```python
from build123d import *

# Parameters (mm, degrees)
F0_W     = 127
F0_H     = 85.5306185286
F1_DEPTH = 254
F2_W     = 44.157743454
F2_H     = 12.9875717685
F3_DEPTH = 76.2
F4_W     = 12.6961972564
F4_H     = 7.905177772
F5_DEPTH = 12.7
F6_W     = 9.1298371553
F6_H     = 11.8159283884
F6_W_2   = 8.5927993059
F6_H_2   = 6.6836136393
F6_W_3   = 35.9823405743
F7_DEPTH = 76.2


with BuildPart() as f1:
    # F0 (on Front) → F1 (new body)
    with BuildSketch(Plane.XZ):
        with Locations((-1.4842953533, -1.855365932)):
            Rectangle(F0_W, F0_H)
    extrude(amount=F1_DEPTH)

    # F2 (on Right) → F3 (join)
    with BuildSketch(Plane.YZ):
        Polygon((-157.0569574833, 18.924748525), (-212.3468965292, 18.924748525), (-212.3468965292, -15.9561578184), (-168.9313054085, -15.9561578184), (-168.9313054085, 0), (-157.0569574833, 0), align=None)
        Polygon((-108.4463298321, 0), (-157.0569574833, 18.924748525), (-157.0569574833, 0), align=None)
        Polygon((-168.9313054085, -15.9561578184), (-212.3468965292, -15.9561578184), (-168.9313054085, -32.6544642448), align=None)
        Polygon((-108.4463298321, 0), (-157.0569574833, 0), (-157.0569574833, -15.9561578184), (-168.9313054085, -15.9561578184), (-168.9313054085, -32.6544642448), (-108.4463298321, -32.6544642448), (-108.4463298321, -21.8933336437), (-116.9810146093, -21.8933336437), (-116.9810146093, -8.9057618752), (-108.4463298321, -8.9057618752), align=None)
        Polygon((-64.2885863781, -8.9057618752), (-108.4463298321, 0), (-108.4463298321, -8.9057618752), align=None)
        with Locations((-86.3674581051, -15.3995477594)):
            Rectangle(F2_W, F2_H)
        Polygon((-108.4463298321, -21.8933336437), (-108.4463298321, -32.6544642448), (-64.2885863781, -21.8933336437), align=None)
    extrude(amount=F3_DEPTH)

    # F4 (on Front) → F5 (join)
    with BuildSketch(Plane.XZ):
        Polygon((-24.3036681507, 11.0724206409), (-24.1946410388, 11.0193416476), (11.4984409884, 11.0193416476), (11.4984409884, 25.6319474429), align=None)
        Polygon((11.4984409884, 11.0193416476), (-24.1946410388, 11.0193416476), (-24.1946410388, 9.8215872422), (-16.5290106088, 9.8215872422), (-16.5290106088, 2.1559579764), (-24.1946410388, 2.1559579764), (-24.1946410388, -17.2476638108), (-18.684970215, -17.2476638108), (-7.1865268983, -17.2476638108), (-7.1865268983, -10.779789649), (19.6431726217, -10.779789649), (19.6431726217, 0), (11.4984409884, 0), align=None)
        Polygon((-24.1946410388, 9.8215872422), (-24.1946410388, 11.0193416476), (-24.3036681507, 11.0724206409), (-42.400509119, 19.8827255517), (-42.400509119, 9.8215872422), align=None)
        Polygon((11.4984409884, 25.6319474429), (11.4984409884, 11.0193416476), (19.6431726217, 11.0193416476), (19.6431726217, 0), (48.6288368702, 0), (48.6288368702, 25.6319474429), align=None)
        Polygon((-24.1946410388, 2.1559579764), (-24.1946410388, 9.8215872422), (-42.400509119, 9.8215872422), (-42.400509119, 7.186527364), (-45.2751219273, 7.186527364), (-45.2751219273, 2.1559579764), (-41.9214069843, 2.1559579764), (-41.9214069843, 4.072365351), (-29.4647607952, 4.072365351), (-29.4647607952, 2.1559579764), align=None)
        Polygon((-24.1946410388, -17.2476638108), (-24.1946410388, 2.1559579764), (-29.4647607952, 2.1559579764), (-29.4647607952, -4.3119159527), align=None)
        Polygon((-45.2751219273, 9.8215872422), (-42.400509119, 9.8215872422), (-42.400509119, 19.8827255517), (-57.9713173211, 19.8827255517), (-57.9713173211, 7.186527364), (-45.2751219273, 7.186527364), align=None)
        Polygon((48.6288368702, 0), (19.6431726217, 0), (19.6431726217, -10.779789649), (31.6207185388, -10.779789649), (31.6207185388, -5.5096708238), (47.6706326008, -5.5096708238), align=None)
        Polygon((-41.9214069843, -12.6961972564), (-24.1946410388, -17.2476638108), (-29.4647607952, -4.3119159527), (-29.4647607952, -12.6961972564), align=None)
        Polygon((-29.4647607952, -4.3119159527), (-29.4647607952, 2.1559579764), (-41.9214069843, 2.1559579764), (-41.9214069843, -12.6961972564), (-29.4647607952, -12.6961972564), align=None)
        Polygon((31.6207185388, -10.779789649), (19.6431726217, -10.779789649), (19.6431726217, -17.2476638108), (-7.1865268983, -17.2476638108), (-7.1865268983, -32.3393717408), (9.5820333809, -32.3393717408), (9.5820333809, -25.3923945129), (22.2782306373, -25.3923945129), (22.2782306373, -32.3393717408), (29.2252078652, -32.3393717408), (35.6930866838, -32.3393717408), (35.6930866838, -24.6737431735), (31.6207185388, -24.6737431735), align=None)
        Polygon((-7.1865268983, -17.2476638108), (-18.684970215, -17.2476638108), (-7.1865268983, -32.3393717408), align=None)
        Polygon((-45.2751219273, 2.1559579764), (-41.9214069843, -12.6961972564), (-41.9214069843, 2.1559579764), align=None)
        Polygon((-45.2751219273, 2.1559579764), (-45.2751219273, 7.186527364), (-57.9713173211, 7.186527364), align=None)
        Polygon((31.6207185388, -5.5096708238), (31.6207185388, -10.779789649), (35.6930866838, -10.779789649), (35.6930866838, -24.6737431735), (47.6706326008, -24.6737431735), (47.6706326008, -5.5096708238), align=None)
        Polygon((9.5820333809, -32.3393717408), (-7.1865268983, -32.3393717408), (9.5820333809, -40.2445495129), align=None)
        Polygon((35.6930866838, -32.3393717408), (47.6706326008, -24.6737431735), (35.6930866838, -24.6737431735), align=None)
        with Locations((15.9301320091, -36.2919606268)):
            Rectangle(F4_W, F4_H)
        Polygon((29.2252078652, -32.3393717408), (22.2782306373, -32.3393717408), (22.2782306373, -40.2445495129), align=None)
    extrude(amount=-F5_DEPTH)

    # F6 (on Right) → F7 (join)
    with BuildSketch(Plane.YZ):
        Polygon((-38.9934703708, -82.4129879475), (-38.9934703708, 11.0402805731), (-61.0125139356, 11.0402805731), (-61.0125139356, -6.6836136393), (-52.4197183549, -6.6836136393), (-52.4197183549, -29.7783855349), (-61.0125139356, -29.7783855349), (-61.0125139356, -82.4129879475), align=None)
        Polygon((-18.666213934, -19.4484525669), (-38.9934703708, 11.0402805731), (-38.9934703708, -82.4129879475), align=None)
        Polygon((-61.0125139356, 11.0402805731), (-38.9934703708, 11.0402805731), (-8.3816275001, 31.4496159554), align=None)
        Polygon((-61.0125139356, -6.6836136393), (-61.0125139356, 11.0402805731), (-137.8106474876, -6.6836136393), align=None)
        Polygon((-61.0125139356, -29.7783855349), (-61.0125139356, -6.6836136393), (-137.8106474876, -6.6836136393), (-137.8106474876, -18.4995420277), (-146.940484643, -18.4995420277), (-146.940484643, -29.7783855349), align=None)
        with Locations((-142.3755660653, -12.5915778335)):
            Rectangle(F6_W, F6_H)
        Polygon((-146.940484643, -6.6836136393), (-137.8106474876, -6.6836136393), (-137.8106474876, 31.9867022336), (-189.9044811726, 31.9867022336), (-189.9044811726, 0), (-181.3116818666, 0), (-181.3116818666, -6.6836136393), (-189.9044811726, -6.6836136393), (-189.9044811726, -17.2098011525), (-185.4956773803, -18.4995420277), (-146.940484643, -18.4995420277), align=None)
        Polygon((-146.940484643, -29.7783855349), (-61.0125139356, -82.4129879475), (-61.0125139356, -29.7783855349), align=None)
        Polygon((-185.4956773803, -18.4995420277), (-146.940484643, -29.7783855349), (-146.940484643, -18.4995420277), align=None)
        Polygon((-189.9044811726, -18.4995420277), (-185.4956773803, -18.4995420277), (-189.9044811726, -17.2098011525), align=None)
        with Locations((-185.6080815196, -3.3418068197)):
            Rectangle(F6_W_2, F6_H_2)
        with Locations((-207.8956514597, -3.3418068197)):
            Rectangle(F6_W_3, F6_H_2)
        Polygon((-225.8868217468, -6.6836136393), (-189.9044811726, -17.2098011525), (-189.9044811726, -6.6836136393), align=None)
    extrude(amount=F7_DEPTH)


solid = f1.part
```
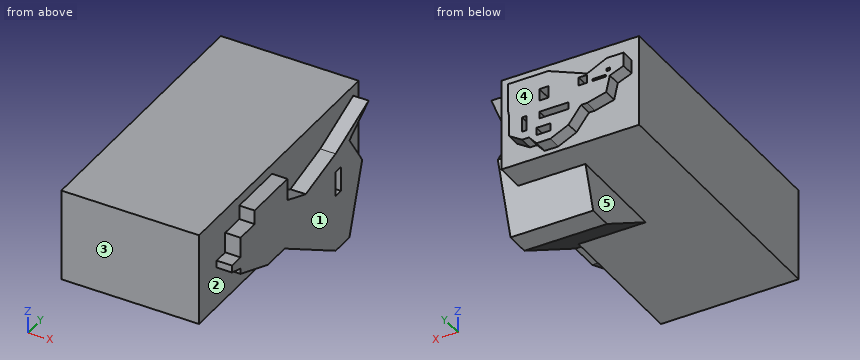
Model file for the job. Use its own axes, mm. Face numbers are marked on the shaded views. A direction names the side the tool comes from. Give positions to 0.01 mm unless a question says otherwise; leave off trailing zeros. Order: outer loops, then holes, each group sorted by start corner. A loop starts at its lowest first (then second) coordinate and runs counter-clockwise, first axis right, second up.
1) Pin check, flat tips, straight feed: pin 1 (10 mm diameter, centred on x = 18.5, y = 8.5, fed in from +Z); pin 2 (6 mm diameter, centred on x = -19.5, y = 8.5, fed in from -Z); pin 3 (11 mm diameter, centred on x = 71, y = -219, fed in from +Z). Stop position of each tip, or through.
2) 3-axis set-ups, long thin cutter, end or side, ignore diameter. For the marked faces 4 and 5: which of +Z, -Z, +X, -X, +Y, -Y reach the whole face in a straight line?
3) Mould opens along Y. For the marked faces 1, 2 and 3 say: +Y half, -Y half, draft (parallel to the pull), parting line (faces both ways), or undercut.
4) Saw through at C-C, the plane x = 42. Write the cut outline in (y, z).
5) Wall check: probe 1 along Z at (x, y) = (58, -141); probe 2 along Y at (x, z) = (8, 35); probe 3 along X at (y, z) = (-234.5, -7). Give the ranges that are in metal, low to high.
6) Saw through at B-B, the plane y = -197. Write the cut outline in (x, z).
7) Saw through at A-A, the plane x = 59. Write the cut outline in (y, z).
8) Saw through at D-D, the plane y = -229. Write the cut outline in (x, z).
Computed:
1. pin 1: stops at z = 25.63
1. pin 2: stops at z = -20.12
1. pin 3: stops at z = 0
2. face 4: +Z, -Z, +X, -X, +Y
2. face 5: -Z, -X, +Y, -Y
3. face 1: draft
3. face 2: undercut
3. face 3: -Y half
4. outline: (-254, -44.62) - (-122.71, -44.62) - (-61.01, -82.41) - (-38.99, -82.41) - (-26.79, -44.62) - (0, -44.62) - (0, -28.3) - (12.7, -28.3) - (12.7, 25.63) - (0, 25.63) - (0, 40.91) - (-254, 40.91) - close
5. probe 1: z = -44.62 to 40.91
5. probe 2: y = -254 to 0
5. probe 3: x = -64.98 to 62.02
6. outline: (-64.98, -44.62) - (62.02, -44.62) - (62.02, -21.86) - (76.2, -21.86) - (76.2, 18.92) - (62.02, 18.92) - (62.02, 40.91) - (-64.98, 40.91) - close
7. outline: (-254, -44.62) - (-122.71, -44.62) - (-61.01, -82.41) - (-38.99, -82.41) - (-26.79, -44.62) - (0, -44.62) - (0, 40.91) - (-254, 40.91) - close
8. outline: (-64.98, -44.62) - (62.02, -44.62) - (62.02, 40.91) - (-64.98, 40.91) - close
